```python
from build123d import *

# Parameters (mm, degrees)
SKETCH1_R           = 45.8343
SKETCH1_R_2         = 34.8869
BOSS_EXTRUDE1_DEPTH = 12.7
CUT_EXTRUDE1_START  = -6.35
CUT_EXTRUDE1_DEPTH  = 6.35
CIRPATTERN1_COUNT   = 4


with BuildPart() as part:
    # Sketch1 → Boss-Extrude1 (new body)
    with BuildSketch(Plane(origin=(0, 0, 0), x_dir=(1, 0, 0), z_dir=(0, 1, 0))):
        with Locations(Location((0, 0, 0), (0, 0, 270))):
            Circle(SKETCH1_R)
        with Locations(Location((0, 0, 0), (0, 0, 270))):
            Circle(SKETCH1_R_2, mode=Mode.SUBTRACT)
    extrude(amount=BOSS_EXTRUDE1_DEPTH)

    # Sketch2 → Cut-Extrude1 (cut)
    with BuildSketch(Plane(origin=(0, 12.7, 0), x_dir=(1, 0, 0), z_dir=(0, 1, 0)).offset(CUT_EXTRUDE1_START)):
        with BuildLine():
            Line((6.35, 34.304129367), (6.35, 38.6969))
            ThreePointArc((6.35, 38.6969), (5.606051224, 40.492951224), (3.81, 41.2369))
            Line((3.81, 41.2369), (-3.81, 41.2369))
            ThreePointArc((-3.81, 41.2369), (-5.606051224, 40.492951224), (-6.35, 38.6969))
            Line((-6.35, 38.6969), (-6.35, 34.304129367))
            ThreePointArc((-6.35, 34.304129367), (0, 34.8869), (6.35, 34.304129367))
        make_face()
    cut_extrude1 = extrude(amount=CUT_EXTRUDE1_DEPTH, mode=Mode.SUBTRACT)

    # CirPattern1: Cut-Extrude1 ×4 about axis
    cirpattern1_axis = Axis((0, 0, 0), (0, 1, 0))
    for i in range(1, CIRPATTERN1_COUNT):
        add(cut_extrude1.rotate(cirpattern1_axis, i * 360 / CIRPATTERN1_COUNT), mode=Mode.SUBTRACT)


solid = part.part
```
Here's how the part is built. I have some questions about the finished solid (model axes, mm). A direction names the side the tool comes from. Round coordinates to 2 decimals unless told otherwise and drop trailing zeros. Write each loop counter-clockwise with the first axis right and the second up, starting at its lowest first coordinate (ties: lowest second). Pieces come first, ordered by that corner, then holes.
Q1. If we section it at A-A on z = 0: Write out the boundary of the cut face in (x, y), plus the area to 3 significant figures.
Q2. If we section it at C-C on y = 9: Write out the boundary of the cut face in (x, z).
Q3. If we section it at D-D on z = -26.5: Write out the boundary of the cut face in (x, y).
Q4. If we section it at B-B on x = 0: Write out the boundary of the cut face in (y, z), plus the area to 3 significant figures.
Q5. Please list where these lines run through material, in increasing order: probe 1 along X at (y, z) = (5, 0); probe 2 along Z at (x, y) = (-40, 11.25).
Q6. If we mould it in two halves opening along Z, with no side actions, what happens to faces 3 (the flat face through (-34, 0, -10)), 4 (the cylindrical face through (5.6, 9.5, -40.5))? For each: +Z half, -Z half, draft (parallel to the pull), parting line (faces both ways), or undercut.
Q7. Which directions (+Z, -Z, +X, -X, +Y, -Y) give clear straight access to the entire face, cutting with the end or side of a thin tool? Please do faces 1 (the cylindrical face through (-13.362, 6.261, 32.227)), 2 (the flat face through (0, 9, 41.237)).
Q8. Will these pins go through, and if not, where does the flat tip stop? P1, Ø1.3, axis at x = 37.5, y = 8, coming from the -Z side; P2, Ø5, axis at x = -0.5, y = 9.5, coming from the +Z side; P3, Ø3.5, axis at y = 9.5, z = 36, coming from the +X side; P4, Ø2, axis at y = 10.5, z = 16, coming from the -X side.
Answer below:
1. outline: (-45.83, 0) - (-34.89, 0) - (-34.89, 6.35) - (-41.24, 6.35) - (-41.24, 12.7) - (-45.83, 12.7) - close; (34.89, 0) - (45.83, 0) - (45.83, 12.7) - (41.24, 12.7) - (41.24, 6.35) - (34.89, 6.35) - close
1. area: 197 mm2
2. outline: circle Ø91.67 at (0, 0); hole (-41.24, -3.81) arc R2.54 ccw to (-38.7, -6.35) - (-34.3, -6.35) arc R34.89 ccw to (-6.35, -34.3) - (-6.35, -38.7) arc R2.54 ccw to (-3.81, -41.24) - (3.81, -41.24) arc R2.54 ccw to (6.35, -38.7) - (6.35, -34.3) arc R34.89 ccw to (34.3, -6.35) - (38.7, -6.35) arc R2.54 ccw to (41.24, -3.81) - (41.24, 3.81) arc R2.54 ccw to (38.7, 6.35) - (34.3, 6.35) arc R34.89 ccw to (6.35, 34.3) - (6.35, 38.7) arc R2.54 ccw to (3.81, 41.24) - (-3.81, 41.24) arc R2.54 ccw to (-6.35, 38.7) - (-6.35, 34.3) arc R34.89 ccw to (-34.3, 6.35) - (-38.7, 6.35) arc R2.54 ccw to (-41.24, 3.81) - close
3. outline: (-37.4, 0) - (-22.69, 0) - (-22.69, 12.7) - (-37.4, 12.7) - close; (22.69, 0) - (37.4, 0) - (37.4, 12.7) - (22.69, 12.7) - close
4. outline: (0, -45.83) - (12.7, -45.83) - (12.7, -41.24) - (6.35, -41.24) - (6.35, -34.89) - (0, -34.89) - close; (0, 34.89) - (6.35, 34.89) - (6.35, 41.24) - (12.7, 41.24) - (12.7, 45.83) - (0, 45.83) - close
4. area: 197 mm2
5. probe 1: x = -45.83 to -34.89, 34.89 to 45.83
5. probe 2: z = -22.38 to -5.99, 5.99 to 22.38
6. face 3: draft
6. face 4: undercut
7. face 1: +Y, -Y
7. face 2: +Y
8. P1: stops at z = -27.26
8. P2: stops at z = 45.83
8. P3: stops at x = 30.46
8. P4: stops at x = -43.31
